from build123d import *

# Parameters (mm, degrees)
EXTRUDE_1_DEPTH     = 6
CUT_EXTRUDE_1_DEPTH = 4
SKETCH_3_R          = 1.72
EXTRUDE_2_DEPTH     = 5.63
EXTRUDE_5_REACH     = 16.5


with BuildPart() as part:
    # 草图1 → 凸台-拉伸1 (new body)
    with BuildSketch(Plane.XY):
        with BuildLine():
            Line((4.5, 0), (4.5, -10))
            Line((4.5, -10), (3, -10))
            Line((3, -10), (3, -6.52))
            ThreePointArc((3, -6.52), (1.968245837, -4.77), (3, -3.02))
            Line((3, -3.02), (3, -1.92))
            Line((3, -1.92), (-3, -1.92))
            Line((-3, -1.92), (-3, -3.02))
            ThreePointArc((-3, -3.02), (-1.968245837, -4.77), (-3, -6.52))
            Line((-3, -6.52), (-3, -10))
            Line((-3, -10), (-4.5, -10))
            Line((-4.5, -10), (-4.5, 0))
            ThreePointArc((-4.5, 0), (0, 4.5), (4.5, 0))
        make_face()
    extrude(amount=EXTRUDE_1_DEPTH)

    # 草图2 → 切除-拉伸1 (cut)
    with BuildSketch(Plane.XY.offset(6)):
        with BuildLine():
            Line((3, 0), (-3, 0))
            ThreePointArc((-3, 0), (0, 3), (3, 0))
        make_face()
    extrude(amount=-CUT_EXTRUDE_1_DEPTH, mode=Mode.SUBTRACT)

    # 草图3 → 凸台-拉伸2 (add)
    with BuildSketch(Plane(origin=(0, 0, 0), x_dir=(-1, 0, 0), z_dir=(0, 0, -1))):
        with Locations((0, 2)):
            Circle(SKETCH_3_R)
    extrude(amount=EXTRUDE_2_DEPTH)

    # 草图4 → 凸台-拉伸5 (add, up to next)
    with BuildSketch(Plane.XZ.offset(10), mode=Mode.PRIVATE) as extrude_5_sk1:
        with BuildLine():
            Line((-3, 0), (-3, 6))
            Line((-3, 6), (-2.5, 5))
            Line((-2.5, 5), (-2.5, 4.5))
            ThreePointArc((-2.5, 4.5), (-2.757359313, 3), (-2.5, 1.5))
            Line((-2.5, 1.5), (-2.5, 1))
            Line((-2.5, 1), (-3, 0))
        make_face()
    extrude_5_tool1 = extrude(extrude_5_sk1.sketch, amount=-EXTRUDE_5_REACH, mode=Mode.PRIVATE) - part.part
    add(extrude_5_tool1.solids().sort_by_distance((-2.809362, -10, 3))[0])
    # 草图4 → 凸台-拉伸5 (add, up to next)
    with BuildSketch(Plane.XZ.offset(10), mode=Mode.PRIVATE) as extrude_5_sk2:
        with BuildLine():
            Line((2.5, 5), (2.5, 4.5))
            ThreePointArc((2.5, 4.5), (2.757359313, 3), (2.5, 1.5))
            Line((2.5, 1.5), (2.5, 1))
            Line((2.5, 1), (3, 0))
            Line((3, 0), (3, 6))
            Line((3, 6), (2.5, 5))
        make_face()
    extrude_5_tool2 = extrude(extrude_5_sk2.sketch, amount=-EXTRUDE_5_REACH, mode=Mode.PRIVATE) - part.part
    add(extrude_5_tool2.solids().sort_by_distance((2.809362, -10, 3))[0])


solid = part.part
Here's how the part is built. I have some questions about the finished solid (model axes, mm). A direction names the side the tool comes from. Round coordinates to 2 decimals unless told otherwise and drop trailing zeros. Order: outer loops, then holes, each group sorted by start corner. A loop starts at its lowest first (then second) coordinate and runs counter-clockwise, first axis right, second up. Notation, with made-up numbers: (87.5, -29) -> (118.5, -29) arc R11 ccw to (118.5, -13) -> close; hole circle Ø7 at (27.25, 16). An arc over 180 degrees is marked (long way). Use CSV: the item, a comma, the result in double quotes.
1. I want a section at B-B on x = 0. List the corners of the cut face in (y, z) for me.
Recorded:
outline,"(-1.92, 0) -> (0.28, 0) -> (0.28, -5.63) -> (3.72, -5.63) -> (3.72, 0) -> (4.5, 0) -> (4.5, 6) -> (3, 6) -> (3, 2) -> (0, 2) -> (0, 6) -> (-1.92, 6) -> close"
2. I want a section at D-D on y = 2.5. List the corners of the cut face in (x, z) for me, and give its area (3 significant figures).
Recorded:
outline,"(-3.74, 0) -> (-1.65, 0) -> (-1.65, -5.63) -> (1.65, -5.63) -> (1.65, 0) -> (3.74, 0) -> (3.74, 6) -> (1.66, 6) -> (1.66, 2) -> (-1.66, 2) -> (-1.66, 6) -> (-3.74, 6) -> close"
area,"50.2 mm2"
3. Which directions (+Z, -Z, +X, -X, +Y, -Y) give clear straight access to the entire face, cutting with the end or side of a thin tool? Please do faces 4 (the face through (2.746, -8.091, 0.507)), 5 (the face through (0, 1, 2)), 6 (the face through (-3, -2.5, 3)).
Recorded:
face 4,"-Z, -Y"
face 5,"+Z"
face 6,"+Z, -Z"
4. I need wall thicknesses on line 1 along Y through (x, z) = (2.75, 5); line 2 along Z through (x, y) = (-1.75, -1); line 3 along X through (y, z) = (-7.25, 1.5). Which ranges of each line are inside material? Lowest first, please.
Recorded:
line 1,"y = -10 to -3.18, -1.92 to 0, 1.2 to 3.56"
line 2,"z = 0 to 6"
line 3,"x = -4.5 to -2.5, 2.5 to 4.5"
5. I want a section at A-A on y = -8.25. List the corners of the cut face in (x, z) for me.
Recorded:
outline,"(-4.5, 0) -> (-3, 0) -> (-2.5, 1) -> (-2.5, 1.5) arc R4.5 cw to (-2.5, 4.5) -> (-2.5, 5) -> (-3, 6) -> (-4.5, 6) -> close; (2.5, 1) -> (3, 0) -> (4.5, 0) -> (4.5, 6) -> (3, 6) -> (2.5, 5) -> (2.5, 4.5) arc R4.5 cw to (2.5, 1.5) -> close"
6. I'm going to push flat-ended pins straight in: P1, Ø2, axis at x = 1, z = 5, coming from the +Y side; P2, Ø3, axis at x = 0, z = 2, coming from the -Y side; P3, Ø1, axis at x = 2.5, y = -4.5, coming from the -Z side. Where does each tip first touch, or does it pass through?
Recorded:
P1,"stops at y = 4.5"
P2,"stops at y = -1.92"
P3,"stops at z = 0"
7. Thinking about a two-plate mould opening in Z: for faces 1 (the face through (0, 0, 4)), 2 (the face through (-2.757, -8.091, 3.021)), 3 (the face through (-2.754, -8.091, 5.507)), which applies, pulls with the +Z half, pulls with the -Z half, needs draft (parallel to the pull), parting line crosses it, or undercut?
Recorded:
face 1,"needs draft"
face 2,"undercut"
face 3,"pulls with the +Z half"
8. I want a section at C-C on z = -0.75. List the corners of the cut face in (x, y) for me, and give its area (3 significant figures).
Recorded:
outline,"circle Ø3.44 at (0, 2)"
area,"9.29 mm2"
